Design review of the part built by this model. Coordinates are the model's own, in mm. Give positions to 0.01 mm unless a question says otherwise; leave off trailing zeros. Order: outer loops, then holes, each group sorted by start corner. A loop starts at its lowest first (then second) coordinate and runs counter-clockwise, first axis right, second up. Notation, with made-up numbers: M 54,29.25 L 91,29.25 A27 cw 91,65.25 Z; hole C 54.5,19.25 d4. An arc over 180 degrees is marked long. Answer as a JSON object with one key per item and string values.
from build123d import *

# Parameters (mm, degrees)
SKETCH_1_R          = 2.2
EXTRUDE_1_DEPTH     = 5
SKETCH_2_W          = 410
SKETCH_2_H          = 226.105378696
CUT_EXTRUDE_2_DEPTH = 5
SKETCH_4_W          = 410
SKETCH_4_H          = 19.486670542
EXTRUDE_3_DEPTH     = 5


with BuildPart() as part:
    # 草图1 → 凸台-拉伸1 (new body)
    with BuildSketch(Plane.XY):
        Polygon((-200, 150), (200, 150), (200, 110), (205, 110), (205, 70), (200, 70), (200, 30), (205, 30), (205, -30), (200, -30), (200, -70), (205, -70), (205, -110), (200, -110), (200, -150), (160, -150), (160, -155), (120, -155), (120, -150), (80, -150), (80, -155), (40, -155), (40, -150), (-40, -150), (-40, -155), (-80, -155), (-80, -150), (-120, -150), (-120, -155), (-160, -155), (-160, -150), (-200, -150), (-200, -110), (-205, -110), (-205, -70), (-200, -70), (-200, -30), (-205, -30), (-205, 30), (-200, 30), (-200, 70), (-205, 70), (-205, 110), (-200, 110), align=None)
        with Locations((-140, -140)):
            Circle(SKETCH_1_R, mode=Mode.SUBTRACT)
        with Locations((-100, -140)):
            Circle(SKETCH_1_R, mode=Mode.SUBTRACT)
        with Locations((-60, -140)):
            Circle(SKETCH_1_R, mode=Mode.SUBTRACT)
        with Locations((-20, -140)):
            Circle(SKETCH_1_R, mode=Mode.SUBTRACT)
        with Locations((20, -140)):
            Circle(SKETCH_1_R, mode=Mode.SUBTRACT)
        with Locations((60, -140)):
            Circle(SKETCH_1_R, mode=Mode.SUBTRACT)
        with Locations((100, -140)):
            Circle(SKETCH_1_R, mode=Mode.SUBTRACT)
        with Locations((140, -140)):
            Circle(SKETCH_1_R, mode=Mode.SUBTRACT)
        with Locations((-190, 110)):
            Circle(SKETCH_1_R, mode=Mode.SUBTRACT)
        with Locations((-190, 70)):
            Circle(SKETCH_1_R, mode=Mode.SUBTRACT)
        with Locations((-190, 30)):
            Circle(SKETCH_1_R, mode=Mode.SUBTRACT)
        with Locations((-190, -30)):
            Circle(SKETCH_1_R, mode=Mode.SUBTRACT)
        with Locations((-190, -70)):
            Circle(SKETCH_1_R, mode=Mode.SUBTRACT)
        with Locations((-190, -110)):
            Circle(SKETCH_1_R, mode=Mode.SUBTRACT)
        with Locations((190, -110)):
            Circle(SKETCH_1_R, mode=Mode.SUBTRACT)
        with Locations((190, -70)):
            Circle(SKETCH_1_R, mode=Mode.SUBTRACT)
        with Locations((190, -30)):
            Circle(SKETCH_1_R, mode=Mode.SUBTRACT)
        with Locations((190, 30)):
            Circle(SKETCH_1_R, mode=Mode.SUBTRACT)
        with Locations((190, 70)):
            Circle(SKETCH_1_R, mode=Mode.SUBTRACT)
        with Locations((190, 110)):
            Circle(SKETCH_1_R, mode=Mode.SUBTRACT)
    extrude(amount=EXTRUDE_1_DEPTH)

    # 草图2 → 切除-拉伸2 (cut)
    with BuildSketch(Plane.XY.offset(5)):
        with Locations((0, 43.052689348)):
            Rectangle(SKETCH_2_W, SKETCH_2_H)
    extrude(amount=-CUT_EXTRUDE_2_DEPTH, mode=Mode.SUBTRACT)

    # 草图4 → 凸台-拉伸3 (add)
    with BuildSketch(Plane.XY.offset(5)):
        with Locations((0, -79.743335271)):
            Rectangle(SKETCH_4_W, SKETCH_4_H)
    extrude(amount=-EXTRUDE_3_DEPTH)


solid = part.part
(1) We need section B-B (x = -114.5). Write out the cut boundary in (y, z).
Checked values:
{"outline": "M -150,0 L -70,0 L -70,5 L -150,5 Z"}
(2) We need section A-A (z = 4.2). Count the separate pieces of the cut face and the enclosed holes in it, plus the area to 3 significant figures.
Checked values:
{"separate pieces": "1", "enclosed holes": "10", "area": "33,000 mm^2"}
(3) To check wall thickness, follow L1, parallel to Y at x = 60, z = 2.95; L2, parallel to Y at x = 100, z = 1; L3, parallel to X at y = -123, z = 3.5. State the ranges of each line that lie inside material, in increasing order. Write a range as from..to.
Checked values:
{"L1": "y = -155..-142.2, -137.8..-70", "L2": "y = -150..-142.2, -137.8..-70", "L3": "x = -200..200"}
(4) Insertion check: pin 1 (1.5 mm diameter, centred on x = -97, z = 3.5, fed in from -Y); pin 2 (1.5 mm diameter, centred on x = -202.5, z = 2, fed in from -Y); pin 3 (2.5 mm diameter, centred on y = -153.5, z = 3, fed in from +X). Each pin has a flat end and moves straight along its axis. Give the tip position at first contact, or say it passes through.
Checked values:
{"pin 1": "stops at y = -150", "pin 2": "stops at y = -110", "pin 3": "stops at x = 160"}
(5) We need section C-C (y = -134). Write out the cut boundary in (x, z), plus the area to 3 significant figures.
Checked values:
{"outline": "M -200,0 L 200,0 L 200,5 L -200,5 Z", "area": "2,000 mm^2"}
